Autodesk Inventor part; units mm, degrees
ref_plane "YZ Plane" through (0, 0, 0) normal (1, 0, 0) x (0, 1, 0)
ref_plane "XZ Plane" through (0, 0, 0) normal (0, 1, 0) x (-1, 0, 0)
ref_plane "XY Plane" through (0, 0, 0) normal (0, 0, 1) x (1, 0, 0)
sketch "Sketch1" plane through (0, 0, 0) normal (0, 0, 1) x (1, 0, 0)
  line L0 (0, 0) -> (50, 0)
  line L1 (50, 0) -> (50, 38)
  line L2 (50, 38) -> (0, 38)
  line L3 (0, 38) -> (0, 0)
  dimension "d0" = 38
  dimension "d3" = 50
extrude "Extrusion1" add sketch "Sketch1" along normal blind 8
sketch "Sketch2" plane through (0, 0, 8) normal (0, 0, 1) x (1, 0, 0)
  line L0 (50, 0) -> (50, 38)
  line L1 (0, 0) -> (50, 0)
  line L2 (50, 38) -> (42, 38)
  line L3 (42, 38) -> (42, 0)
  line L4 (42, 0) -> (50, 0)
  line L5 (50, 0) -> (50, 38)
  dimension "d4" = 8
extrude "Extrusion2" add sketch "Sketch2" along normal blind 42
sketch "Sketch3" plane through (0, 0, 0) normal (0, -1, 0) x (1, 0, 0)
  line L0 (42, 8) -> (42, 50)
  line L1 (42, 30) -> (20, 8)
  line L2 (0, 8) -> (42, 8)
  line L3 (0, 0) -> (50, 0)
  line L4 (50, 0) -> (50, 50)
  dimension "d7" = 30
  dimension "d8" = 30
extrude "Extrusion3" add sketch "Sketch3" against normal up to surface (38 mm away)
sketch "Sketch4" plane through (42, 0, 50) normal (-1, 0, 0) x (0, 0, 1)
  circle A0 centre (-10, 19) radius 4.5
  line L0 (0, 38) -> (0, 0)
  line L1 (-20, 38) -> (0, 38)
  point P0 (-50, 0)
  dimension "d11" = 10
  dimension "d12" = 19
  dimension "d13" = 9
extrude "Extrusion4" cut sketch "Sketch4" against normal through all
sketch "Sketch5" plane through (0, 0, 8) normal (0, 0, 1) x (1, 0, 0)
  circle A0 centre (10, 19) radius 4.5
  line L0 (0, 38) -> (0, 0)
  line L1 (0, 0) -> (20, 0)
  dimension "d16" = 10
  dimension "d17" = 19
  dimension "d18" = 9
extrude "Extrusion5" cut sketch "Sketch5" against normal blind 10
properties part number "KeNhom40"
The model under review builds one solid part; all positions refer to its coordinate system, in mm. A direction names the side the tool comes from. Round coordinates to 2 decimals unless told otherwise and drop trailing zeros. Loops run counter-clockwise (first coordinate to the right, second up) from the corner with the lowest first, then second, coordinate; pieces in that order, holes last. Notation, with made-up numbers: (23, 76.25) -> (72, 76.25) arc R17 cw to (72, 87.25) -> close; hole circle Ø1 at (75.5, 45.25). An arc over 180 degrees is marked (long way). Answer in a Markdown table with one row per item.
1) Wall thickness on line 1 along Y through (x, z) = (10, 6.25); line 2 along Z through (x, y) = (17, 11); line 3 along Z through (x, y) = (32, 8): over which ranges is each line inside the solid? List them lowest first.
Taken from the geometry:
| item | result |
|---|---|
| line 1 | y = 0 to 14.5, 23.5 to 38 |
| line 2 | z = 0 to 8 |
| line 3 | z = 0 to 20 |
2) Consider section D-D, the plane y = 11. Write out the cut boundary in (x, z).
Taken from the geometry:
| item | result |
|---|---|
| outline | (0, 0) -> (50, 0) -> (50, 50) -> (42, 50) -> (42, 30) -> (20, 8) -> (0, 8) -> close |
3) Consider section A-A, the plane y = 19. Write out the cut boundary in (x, z), plus the area to 3 significant figures.
Taken from the geometry:
| item | result |
|---|---|
| outline | (0, 0) -> (5.5, 0) -> (5.5, 8) -> (0, 8) -> close; (14.5, 0) -> (50, 0) -> (50, 35.5) -> (42, 35.5) -> (42, 30) -> (20, 8) -> (14.5, 8) -> close; (42, 44.5) -> (50, 44.5) -> (50, 50) -> (42, 50) -> close |
| area | 834 mm² |
4) For pin 1 Ø8 at (x, y) = (10, 19) entering from +Z (3 decimals); pin 2 Ø10 at (y, z) = (25, 44.5) entering from -X; pin 3 Ø1.5 at (y, z) = (11.5, 19) entering from -X; pin 4 Ø4 at (x, y) = (7.5, 26.5) entering from -Z, all flat-tipped, find the tip position at first contact; note any pin that passes through.
Taken from the geometry:
| item | result |
|---|---|
| pin 1 | passes through |
| pin 2 | stops at x = 42 |
| pin 3 | stops at x = 30.25 |
| pin 4 | stops at z = 0 |
5) Draft analysis for pull direction X (two halves, no side actions). For faces 3 (the flat face through (34, 0, 16)), 4 (the cylindrical face through (12.419, 22.794, 4.056)), 5 (the flat face through (50, 19, 25)), 6 (the flat face through (42, 19, 35)), state which applies: pulls with the +X half, pulls with the -X half, needs draft (parallel to the pull), parting line crosses it, or undercut.
Taken from the geometry:
| item | result |
|---|---|
| face 3 | needs draft |
| face 4 | undercut |
| face 5 | pulls with the +X half |
| face 6 | pulls with the -X half |
6) Consider section B-B, the plane z = 40. Write out the cut boundary in (x, y), plus the area to 3 significant figures.
Taken from the geometry:
| item | result |
|---|---|
| outline | (42, 0) -> (50, 0) -> (50, 14.5) -> (42, 14.5) -> close; (42, 23.5) -> (50, 23.5) -> (50, 38) -> (42, 38) -> close |
| area | 232 mm² |
7) Tool access review of faces 1 (the flat face through (25, 19, 0)), 2 (the flat face through (5, 19, 8)): name each direction out of +Z, -Z, +X, -X, +Y, -Y from which nothing blocks a thin tool from reaching the whole face with its end or side.
Taken from the geometry:
| item | result |
|---|---|
| face 1 | -Z, +X, -X, +Y, -Y |
| face 2 | +Z, -X, +Y, -Y |
8) Consider section C-C, the plane x = 10. Write out the cut boundary in (y, z).
Taken from the geometry:
| item | result |
|---|---|
| outline | (0, 0) -> (14.5, 0) -> (14.5, 8) -> (0, 8) -> close; (23.5, 0) -> (38, 0) -> (38, 8) -> (23.5, 8) -> close |
